Autodesk Inventor part; units mm, degrees
ref_plane "YZ Plane" through (0, 0, 0) normal (1, 0, 0) x (0, 1, 0)
ref_plane "XZ Plane" through (0, 0, 0) normal (0, 1, 0) x (-1, 0, 0)
ref_plane "XY Plane" through (0, 0, 0) normal (0, 0, 1) x (1, 0, 0)
sketch "スケッチ1" plane through (0, 0, 0) normal (0, 0, 1) x (1, 0, 0)
  line L0 (1.5, 1.2) -> (2.5, 1.2)
  line L1 (3, 0.9113) -> (3, -1.2)
  line L2 (3, -1.2) -> (1.5, -1.2)
  line L3 (1.5, -1.2) -> (1.5, 1.2)
  line L4 (0, 1.2) -> (0, -1.2)
  line L5 (2.5, 1.2) -> (3, 0.9113)
  point P0 (0, 0)
  dimension "d0" = 1.2
  dimension "d1" = 2.4
  dimension "d2" = 1.5
  dimension "d3" = 3
  dimension "d4" = 1
  dimension "d5" = 30
revolve "回転1" add sketch "スケッチ1" angle 360 about axis through (0, 1.2, 0) along (0, -1, 0)
sketch "スケッチ2" plane through (0, 1.2, 0) normal (0, 1, 0) x (1, 0, 0)
  circle A0 centre (0, 0) radius 1.5
  line L0 (0, 3) -> (2.5981, 1.5)
  line L1 (2.5981, 1.5) -> (2.5981, -1.5)
  line L2 (2.5981, -1.5) -> (0, -3)
  line L3 (0, -3) -> (-2.5981, -1.5)
  line L4 (-2.5981, -1.5) -> (-2.5981, 1.5)
  line L5 (-2.5981, 1.5) -> (0, 3)
  dimension "d7" = 3
extrude "押し出し1" cut sketch "スケッチ2" against normal blind 2.4 keep common part
thread "ねじ1"
properties material "ステンレス鋼"
The listing builds one solid part. Answer for the finished solid, in the listing's coordinates (mm). Round coordinates to 2 decimals unless told otherwise and drop trailing zeros. Loops run counter-clockwise (first coordinate to the right, second up) from the corner with the lowest first, then second, coordinate; pieces in that order, holes last. Notation, with made-up numbers: (8.25, 22.5) - (59.25, 22.5) arc R5 cw to (59.25, 29.5) - close; hole circle Ø3 at (66, 41.25). An arc over 180 degrees is marked (long way). Use one line per item in the form item = value. Start each with the question number.
1. Consider line 1 (X direction, y = 0.45, z = 0.9); line 2 (Z direction, x = -0.8, y = -0.1); line 3 (Z direction, x = -0.3, y = -1.1). Determine where each line is inside the solid, lowest interval first. Write a range as [from, to].
2. The part is cut by section A-A on z = 0. Determine the outline of the cut face in (x, y), then the cut area to 3 significant figures.
3. For a pull along Z with two mould halves and no side action, classify faces 1 (the face through (-1.32, -0.01, -2.24)), 2 (the face through (2.598, 0, 0)), 3 (the face through (-1.5, 0.02, -0.07)) as pulls with the +Z half, pulls with the -Z half, needs draft (parallel to the pull), parting line crosses it, or undercut.
4. The part is cut by section C-C on y = 1. Determine the outline of the cut face in (x, z).
5. Given pin 1 Ø1 at (x, y) = (-1.5, -0.5) entering from -Z; pin 2 Ø1.8 at (x, z) = (0, 0) entering from +Y, each flat-ended and moving along its own axis, determine where each tip first touches the part or whether it passes through.
Geometry check:
q1.line_1 = [-2.6, -1.2], [1.2, 2.6]
q1.line_2 = [-2.54, -1.27], [1.27, 2.54]
q1.line_3 = [-2.83, -1.47], [1.47, 2.83]
q2.outline = (-2.6, -1.2) - (-1.5, -1.2) - (-1.5, 1.2) - (-2.5, 1.2) - (-2.6, 1.14) - close; (1.5, -1.2) - (2.6, -1.2) - (2.6, 1.14) - (2.5, 1.2) - (1.5, 1.2) - close
q2.area = 5.27 mm^2
q3.face_1 = pulls with the -Z half
q3.face_2 = needs draft
q3.face_3 = undercut
q4.outline = (-2.6, -1.16) arc R2.85 ccw to (-2.31, -1.67) - (-0.29, -2.83) arc R2.85 ccw to (0.29, -2.83) - (2.31, -1.67) arc R2.85 ccw to (2.6, -1.16) - (2.6, 1.16) arc R2.85 ccw to (2.31, 1.67) - (0.29, 2.83) arc R2.85 ccw to (-0.29, 2.83) - (-2.31, 1.67) arc R2.85 ccw to (-2.6, 1.16) - close; hole circle Ø3 at (0, 0)
q5.pin_1 = -2.42
q5.pin_2 = through
